Verification items for the finished model (mm, model axes). Round coordinates to 2 decimals unless told otherwise and drop trailing zeros. Order: outer loops, then holes, each group sorted by start corner. A loop starts at its lowest first (then second) coordinate and runs counter-clockwise, first axis right, second up. Notation, with made-up numbers: M 63.25,52.25 L 67.25,52.25 A15 cw 67.25,65.25 Z; hole C 1.5,68 d11. An arc over 180 degrees is marked long. Write item = value, one per line. Start each with the question number.
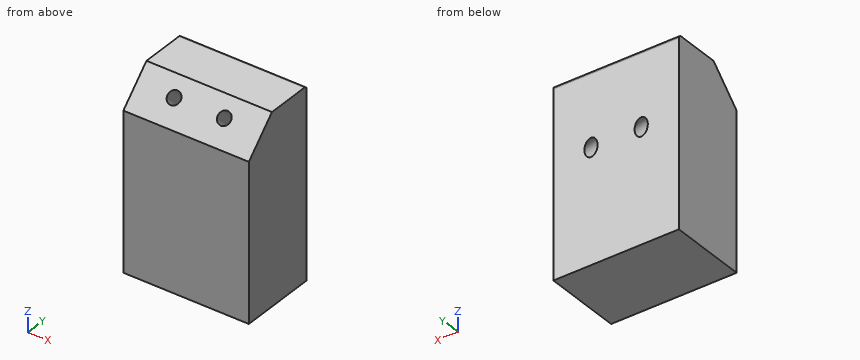
from build123d import *

# Parameters (mm, degrees)
F0_W     = 40
F0_H     = 60
F1_DEPTH = 25
F2_SIZE  = 10
F4_D     = 4.2
F5_R     = 1


with BuildPart() as f1:
    # F0 (on Front) → F1 (new body)
    with BuildSketch(Plane.XZ):
        with Locations((-20, 30)):
            Rectangle(F0_W, F0_H)
    extrude(amount=F1_DEPTH)

    # F2
    f2_edges = [f1.edges().sort_by_distance(p)[0] for p in [
        (-20, -25, 60),
    ]]
    chamfer(f2_edges, length=F2_SIZE)

    # F4 (through all)
    with Locations(Plane(origin=(0, -37.5, 37.5), x_dir=(1, 0, 0), z_dir=(0, -0.7071067812, 0.7071067812))):
        with Locations((-12, 25.6776695297), (-28, 25.6776695297)):
            Hole(F4_D / 2)

    # F5
    f5_edges = [f1.edges().sort_by_distance(p)[0] for p in [
        (-20, 0, 60),
    ]]
    fillet(f5_edges, radius=F5_R)


solid = f1.part
1) Scan lines: probe 1 along Z at (x, y) = (-36.5, -16); probe 2 along Y at (x, z) = (-13.5, 49); probe 3 along Y at (x, z) = (-12.5, 49). Record each from-to range of solid material in increasing order.
2) Cross-section at A-A, the plane x = -15.5. Enter the section's corners in (y, z), then the cut area to 3 significant figures.
3) Gauge pin test, flat end, axial feed: P1, Ø6, axis at x = -21.5, z = 33, coming from the +Y side. Record the tip position at first contact, or that the pin passes through.
4) Cross-section at B-B, the plane y = -22.25. Enter the section's corners in (x, z).
5) Cross-section at C-C, the plane z = 39.5. Give the number of separate pieces and of enclosed holes in the cut face, then the cut area to 3 significant figures.
Geometry results:
q1.probe_1 = 0 to 59
q1.probe_2 = -25 to -14.76, -10.61 to 0
q1.probe_3 = -25 to -15.57, -9.8 to 0
q2.outline = M -25,0 L 0,0 L 0,59 A1 ccw -1,60 L -15,60 L -25,50 Z
q2.area = 1,450 mm^2
q3.P1 = 0
q4.outline = M -40,0 L 0,0 L 0,52.75 L -40,52.75 Z
q5.separate_pieces = 1
q5.enclosed_holes = 2
q5.area = 961 mm^2
